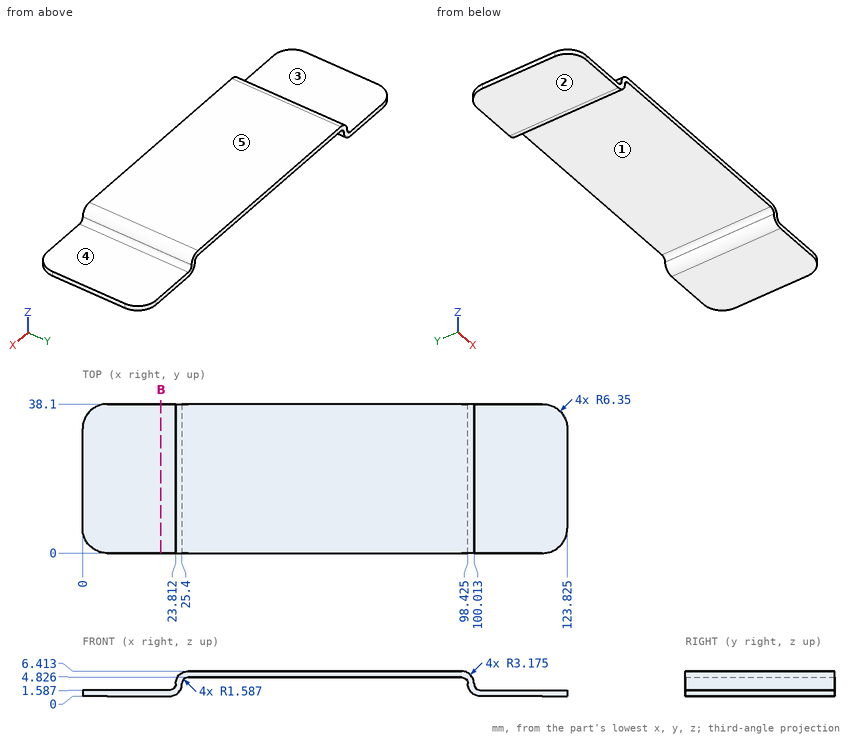
Can you work these out from the drawing? Everything is in mm from the part's minimum corner. A direction names the side the tool comes from. Give positions to 0.01 mm unless a question says otherwise; leave off trailing zeros. Order: outer loops, then holes, each group sorted by start corner. A loop starts at its lowest first (then second) coordinate and runs counter-clockwise, first axis right, second up. Notation, with made-up numbers: M 49.25,-31 L 79.25,-31 A14 cw 79.25,-19 Z; hole C 24,38 d4. An arc over 180 degrees is marked long. Use a Markdown table: item, result. Add a question column.
1. I need wall thicknesses on probe 1 along X at (y, z) = (27.5, 3) (1 decimal); probe 2 along Z at (x, y) = (104.5, 22); probe 3 along Z at (x, y) = (36, 3) (1 decimal). Which ranges of each line are inside material? Lowest first, please. Write a range as from..to.
2. On a 3-axis mill with a long thin cutter (end or side, diameter ignored), from which of +Z, -Z, +X, -X, +Y, -Y can I reach the whole of each face in a straight line? I mean the marked faces 3, 4 and 5. Say none if no direction works.
3. Suppose I cut it at B-B (x = 20). List the corners of the cut face in (y, z) for me.
4. For pin 1 Ø11 at (x, y) = (9, 28.5) entering from +Z; pin 2 Ø3 at (x, z) = (69.5, 3) entering from -Y; pin 3 Ø1.5 at (x, y) = (95, 32) entering from -Z, each with a flat end and sliding along its axis, tell me the tip position at first contact or that it passes through.
5. If we mould it in two halves opening along X, with no side actions, what happens to the marked faces 1 and 2? For each: +X half, -X half, draft (parallel to the pull), parting line (faces both ways), or undercut.
Results list:
| question | item | result |
|---|---|---|
| 1 | probe 1 | x = 23.8..25.4, 98.4..100 |
| 1 | probe 2 | z = 0..1.59 |
| 1 | probe 3 | z = 4.8..6.4 |
| 2 | face 3 | +Z, -X, +Y, -Y |
| 2 | face 4 | +Z, +X, +Y, -Y |
| 2 | face 5 | +Z, +X, -X, +Y, -Y |
| 3 | outline | M 0,0 L 38.1,0 L 38.1,1.59 L 0,1.59 Z |
| 4 | pin 1 | stops at z = 1.59 |
| 4 | pin 2 | passes through |
| 4 | pin 3 | stops at z = 4.83 |
| 5 | face 1 | undercut |
| 5 | face 2 | draft |
